Check sheet for the modelled part. Datum: model origin and axes. Units: mm. Face numbers are marked on the shaded views. A direction names the side the tool comes from. Give positions to 0.01 mm unless a question says otherwise; leave off trailing zeros. Order: outer loops, then holes, each group sorted by start corner. A loop starts at its lowest first (then second) coordinate and runs counter-clockwise, first axis right, second up. Notation, with made-up numbers: (-22.5, -8.75) -> (-5.5, -8.75) arc R22 cw to (-5.5, 7.25) -> close; hole circle Ø1 at (-22.5, 41). An arc over 180 degrees is marked (long way). Write each question's results on one line, items separated by ' | '.
Autodesk Inventor part; units mm, degrees
ref_plane "YZ Plane" through (0, 0, 0) normal (1, 0, 0) x (0, 1, 0)
ref_plane "XZ Plane" through (0, 0, 0) normal (0, 1, 0) x (-1, 0, 0)
ref_plane "XY Plane" through (0, 0, 0) normal (0, 0, 1) x (1, 0, 0)
sketch "Sketch1" plane through (0, 0, 0) normal (0, 1, 0) x (-1, 0, 0)
  line L0 (-10, 10) -> (10, 10)
  line L1 (10, 10) -> (10, -10)
  line L2 (10, -10) -> (-10, -10)
  line L3 (-10, -10) -> (-10, 10)
  line L4 (-10, 10) -> (10, -10) construction
  line L5 (10, 10) -> (-10, -10) construction
  point P0 (0, 0)
extrude "Extrusion1" add sketch "Sketch1" along normal blind 2
sketch "Sketch2" plane through (0, 2, 0) normal (0, 1, 0) x (1, 0, 0)
  line L0 (9, -9) -> (-9, -9)
  line L1 (-9, -9) -> (-9, 9)
  line L2 (-9, 9) -> (9, 9)
  line L3 (9, 9) -> (9, -9)
  line L4 (9, -9) -> (-9, 9) construction
  line L5 (-9, -9) -> (9, 9) construction
  line L6 (10, -10) -> (-10, -10)
  line L7 (-10, -10) -> (-10, 10)
  line L8 (-10, 10) -> (10, 10)
  line L9 (10, 10) -> (10, -10)
  line L10 (10, -10) -> (-10, 10) construction
  line L11 (-10, -10) -> (10, 10) construction
  point P0 (0, 0)
extrude "Extrusion2" add sketch "Sketch2" along normal blind 5
sketch "Sketch3" plane through (0, 2, 0) normal (0, 1, 0) x (1, 0, 0)
  circle A0 centre (0, 0) radius 2.9425
  line L0 (0.626, -2.1935) -> (-0.626, -2.1935)
  line L1 (-0.626, 2.1935) -> (0.626, 2.1935)
  line L2 (-2.1935, 0.626) -> (-2.1935, -0.626)
  line L3 (2.1935, -0.626) -> (2.1935, 0.626)
  line L4 (-0.626, -2.1935) -> (-0.626, -0.626)
  line L5 (-0.626, 0.626) -> (-0.626, 2.1935)
  line L6 (-2.1935, -0.626) -> (-0.626, -0.626)
  line L7 (0.626, -0.626) -> (2.1935, -0.626)
  line L8 (2.1935, 0.626) -> (0.626, 0.626)
  line L9 (-0.626, 0.626) -> (-2.1935, 0.626)
  line L10 (0.626, 2.1935) -> (0.626, 0.626)
  line L11 (0.626, -0.626) -> (0.626, -2.1935)
extrude "Extrusion4" add sketch "Sketch3" along normal blind 3.9
fillet "Fillet1" radius 0.3 4 edges at (-0.626, 3.95, -0.626) (-0.626, 3.95, 0.626) (0.626, 3.95, -0.626) (0.626, 3.95, 0.626)
properties part number "test2"
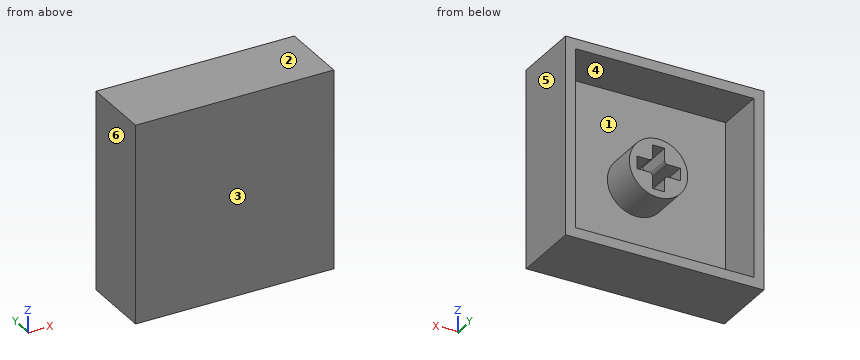
1. Material ranges on probe 1 along Z at (x, y) = (4.75, 5.75); probe 2 along X at (y, z) = (3.5, -1.5), recorded low to high. Write a range as from..to.
Verdict:
probe 1: z = -10..-9, 9..10 | probe 2: x = -10..-9, -2.53..-0.63, 0.63..2.53, 9..10
2. Access from +Z, -Z, +X, -X, +Y, -Y to the whole of each face (thin tool, end or side, straight path). Record for the marked faces 1 and 2.
Verdict:
face 1: +Y | face 2: +Z, +X, -X, +Y, -Y
3. Section check C-C on x = 3.5. Record the cut outline in (y, z), then the cut area to 3 significant figures.
Verdict:
outline: (0, -10) -> (7, -10) -> (7, -9) -> (2, -9) -> (2, 9) -> (7, 9) -> (7, 10) -> (0, 10) -> close | area: 50.0 mm^2
4. Section check D-D on x = 0. Record the cut outline in (y, z), then the cut area to 3 significant figures.
Verdict:
outline: (0, -10) -> (7, -10) -> (7, -9) -> (2, -9) -> (2, -2.94) -> (5.9, -2.94) -> (5.9, -2.19) -> (2, -2.19) -> (2, 2.19) -> (5.9, 2.19) -> (5.9, 2.94) -> (2, 2.94) -> (2, 9) -> (7, 9) -> (7, 10) -> (0, 10) -> close | area: 55.8 mm^2
5. Section check A-A on y = 3.5. Record the cut outline in (x, z) (1 decimal).
Verdict:
outline: (-10, -10) -> (10, -10) -> (10, 10) -> (-10, 10) -> close; circle Ø5.9 at (0, 0); hole (-9, -9) -> (9, -9) -> (9, 9) -> (-9, 9) -> close; hole (-2.2, -0.6) -> (-0.9, -0.6) arc R0.3 cw to (-0.6, -0.9) -> (-0.6, -2.2) -> (0.6, -2.2) -> (0.6, -0.9) arc R0.3 cw to (0.9, -0.6) -> (2.2, -0.6) -> (2.2, 0.6) -> (0.9, 0.6) arc R0.3 cw to (0.6, 0.9) -> (0.6, 2.2) -> (-0.6, 2.2) -> (-0.6, 0.9) arc R0.3 cw to (-0.9, 0.6) -> (-2.2, 0.6) -> close
6. Gauge pin test, flat end, axial feed: pin 1 Ø4.5 at (x, z) = (0.5, -0.5) entering from +Y. Record the tip position at first contact, or that the pin passes through.
Verdict:
pin 1: stops at y = 5.9
7. Mould release check, pull along X, two halves, no side actions. Record for the marked faces 3, 4, 5 and 6: +X half, -X half, draft (parallel to the pull), parting line (faces both ways), or undercut.
Verdict:
face 3: draft | face 4: undercut | face 5: +X half | face 6: -X half
8. Section check B-B on z = 0. Record the cut outline in (x, y).
Verdict:
outline: (-10, 0) -> (10, 0) -> (10, 7) -> (9, 7) -> (9, 2) -> (2.94, 2) -> (2.94, 5.9) -> (2.19, 5.9) -> (2.19, 2) -> (-2.19, 2) -> (-2.19, 5.9) -> (-2.94, 5.9) -> (-2.94, 2) -> (-9, 2) -> (-9, 7) -> (-10, 7) -> close
